Autodesk Inventor part; units mm, degrees
ref_plane "YZ Plane" through (0, 0, 0) normal (1, 0, 0) x (0, 1, 0)
ref_plane "XZ Plane" through (0, 0, 0) normal (0, 1, 0) x (-1, 0, 0)
ref_plane "XY Plane" through (0, 0, 0) normal (0, 0, 1) x (1, 0, 0)
sketch "Sketch1" plane through (0, 0, 0) normal (0, 0, 1) x (1, 0, 0)
  circle A0 centre (0, 0) radius 2.4 construction
  line L0 (-0.8, 2.2627) -> (-0.8, 0.8)
  line L1 (-0.8, 0.8) -> (-2.2627, 0.8)
  line L2 (-2.2627, -0.8) -> (-0.8, -0.8)
  line L3 (-0.8, -0.8) -> (-0.8, -2.2627)
  line L4 (0.8, -2.2627) -> (0.8, -0.8)
  line L5 (0.8, -0.8) -> (2.2627, -0.8)
  line L6 (2.2627, 0.8) -> (0.8, 0.8)
  line L7 (0.8, 0.8) -> (0.8, 2.2627)
  arc A1 (0.8, 2.2627) -> (-0.8, 2.2627) centre (0, 0) ccw
  arc A2 (-2.2627, 0.8) -> (-2.2627, -0.8) centre (0, 0) ccw
  arc A3 (-0.8, -2.2627) -> (0.8, -2.2627) centre (0, 0) ccw
  arc A4 (2.2627, -0.8) -> (2.2627, 0.8) centre (0, 0) ccw
  dimension "d0" = 4.8
  dimension "d1" = 1.6
extrude "Extrusion1" add sketch "Sketch1" along normal mid plane 72
fillet "Fillet1" radius 0.4 8 edges at (0, 2.4, 36) (-2.4, 0, 36) (0, -2.4, 36) (2.4, 0, 36) (2.4, 0, -36) (0, 2.4, -36) (-2.4, 0, -36) (0, -2.4, -36)
equation "\"d0\" = kd"
equation "\"d1\" = axlet"
equation "\"d2\" = 9 * lu"
equation "\"d4\" = tf"
properties part number "60485-LtBluishGray" material "ABS Plastic"
Can you work these out from the model? Positions are in its coordinate system, mm. A direction names the side the tool comes from. Coordinates: 2 decimals unless noted, no trailing zeros. Order: outer loops, then holes, each group sorted by start corner. A loop starts at its lowest first (then second) coordinate and runs counter-clockwise, first axis right, second up. Notation, with made-up numbers: M -26,-32.5 L 26,-32.5 A13 ccw 26,-17.5 Z; hole C 61,69 d6. An arc over 180 degrees is marked long. Write item = value, one per line.
(1) Suppose I cut it at A-A on z = -8.5. Please give me the cut outline in (x, y), plus the area to 3 significant figures.
Results are:
outline = M -2.26,-0.8 L -0.8,-0.8 L -0.8,-2.26 A2.4 ccw 0.8,-2.26 L 0.8,-0.8 L 2.26,-0.8 A2.4 ccw 2.26,0.8 L 0.8,0.8 L 0.8,2.26 A2.4 ccw -0.8,2.26 L -0.8,0.8 L -2.26,0.8 A2.4 ccw Z
area = 12.5 mm2
(2) I need wall thicknesses on line 1 along Y through (x, z) = (-0.9, 29.5); line 2 along X through (y, z) = (-0.4, 7.5). Which ranges of each line are inside material? Lowest first, please. Write a range as [from, to].
Results are:
line_1 = [-0.8, 0.8]
line_2 = [-2.37, 2.37]
(3) For pin 1 Ø0.7 at (x, z) = (-1.5, 15) entering from -Y; pin 2 Ø1.2 at (x, z) = (-1.5, -15) entering from +Y; pin 3 Ø0.7 at (y, z) = (-1.5, -8.5) entering from +X, each with a flat end and sliding along its axis, tell me the tip position at first contact or that it passes through.
Results are:
pin_1 = -0.8
pin_2 = 0.8
pin_3 = 0.8
(4) For faces 1 (the face through (-2, 0.8, -1)), 2 (the face through (-0.8, -2, -1)), 3 (the face through (2, 0.8, -1)), 4 (the face through (2, -0.8, -1)), which set-ups out of +Z, -Z, +X, -X, +Y, -Y let a thin tool reach every point of the face, with its end or its side?
Results are:
face_1 = +Z, -Z, -X, +Y
face_2 = +Z, -Z, -X, -Y
face_3 = +Z, -Z, +X, +Y
face_4 = +Z, -Z, +X, -Y
